Design review of the part built by this model. Coordinates are the model's own, in mm. Face numbers are marked on the shaded views. A direction names the side the tool comes from. Coordinates: 2 decimals unless noted, no trailing zeros. Loops run counter-clockwise (first coordinate to the right, second up) from the corner with the lowest first, then second, coordinate; pieces in that order, holes last. Notation, with made-up numbers: M 32,17.25 L 53,17.25 A31 cw 53,49.25 Z; hole C -19.5,47 d9. An arc over 180 degrees is marked long. One line per item, written item: value.
```python
from build123d import *

# Parameters (mm, degrees)
F0_W     = 127
F0_H     = 76.2
F1_DEPTH = 25.4
F2_W     = 25.4
F2_H     = 25.4
F2_R     = 12.7
F3_DEPTH = 2540


with BuildPart() as f1:
    # F0 (on Right) → F1 (new body)
    with BuildSketch(Plane.YZ):
        with Locations((-7.924328, 38.1)):
            Rectangle(F0_W, F0_H)
    extrude(amount=F1_DEPTH)

    # F2 (on face) → F3 (cut)
    with BuildSketch(Plane(origin=(0, 0, 0), x_dir=(0, -1, 0), z_dir=(-1, 0, 0))):
        with Locations((-31.45644, 49.823285)):
            Rectangle(F2_W, F2_H)
        with Locations((29.554684, 46.785511)):
            Circle(F2_R)
    extrude(amount=-F3_DEPTH, mode=Mode.SUBTRACT)


solid = f1.part
```
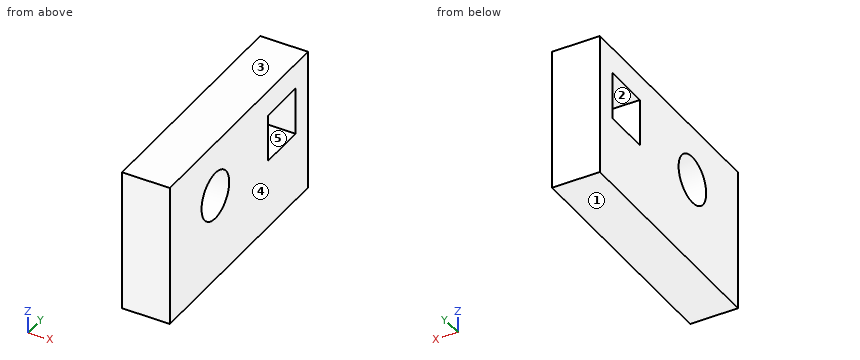
(1) We need section A-A on y = 31. State the section outline as (x, z) points.
Reply:
outline: M 0,0 L 25.4,0 L 25.4,37.12 L 0,37.12 Z; M 0,62.52 L 25.4,62.52 L 25.4,76.2 L 0,76.2 Z
(2) We need section D-D on y = -35. State the section outline as (x, z) points.
Reply:
outline: M 0,0 L 25.4,0 L 25.4,35.31 L 0,35.31 Z; M 0,58.26 L 25.4,58.26 L 25.4,76.2 L 0,76.2 Z
(3) We need section B-B on z = 51. State the section outline as (x, y) points (3 decimals).
Reply:
outline: M 0,-71.424 L 25.4,-71.424 L 25.4,-41.535 L 0,-41.535 Z; M 0,-17.574 L 25.4,-17.574 L 25.4,18.756 L 0,18.756 Z; M 0,44.156 L 25.4,44.156 L 25.4,55.576 L 0,55.576 Z
(4) Tool access review of the marked faces 1 and 2: name each direction out of +Z, -Z, +X, -X, +Y, -Y from which nothing blocks a thin tool from reaching the whole face with its end or side.
Reply:
face 1: -Z, +X, -X, +Y, -Y
face 2: +X, -X
(5) Mouldability with a two-part tool opening along Z and no side actions: class the marked faces 3, 4 and 5 as released by +Z, released by -Z, zero draft, split by the parting line, or undercut.
Reply:
face 3: released by +Z
face 4: zero draft
face 5: undercut
(6) We need section C-C on x = 17. State the section outline as (y, z) points, then the cut area to 3 significant figures.
Reply:
outline: M -71.42,0 L 55.58,0 L 55.58,76.2 L -71.42,76.2 Z; hole C -29.55,46.79 d25.4; hole M 18.76,37.12 L 44.16,37.12 L 44.16,62.52 L 18.76,62.52 Z
area: 8,530 mm2
(7) To check wall thickness, follow line 1 along Y through (x, z) = (7.75, 46.5); line 2 along Z through (x, y) = (17.25, 26); line 3 along Y through (x, z) = (8.75, 38). State the ranges of each line that lie inside material, in increasing order. Write a range as [from, to].
Reply:
line 1: y = [-71.42, -42.25], [-16.86, 18.76], [44.16, 55.58]
line 2: z = [0, 37.12], [62.52, 76.2]
line 3: y = [-71.42, -38.73], [-20.38, 18.76], [44.16, 55.58]
